```python
from build123d import *

# Parameters (mm, degrees)
SKETCH1_R           = 6.5
BOSS_EXTRUDE1_DEPTH = 3.5
SKETCH2_R           = 2
CUT_EXTRUDE1_DEPTH  = 10
CUT_EXTRUDE2_START  = -3.5
CUT_EXTRUDE2_DEPTH  = 1


with BuildPart() as part:
    # Sketch1 → Boss-Extrude1 (new body)
    with BuildSketch(Plane.XY):
        with BuildLine():
            Line((-15, 0), (-22.911315665, -21.736161147))
            ThreePointArc((-22.911315665, -21.736161147), (-25.84024514, -25.553216354), (-30.428856631, -27))
            Line((-30.428856631, -27), (-35, -27))
            Line((-35, -27), (-35, -35))
            Line((-35, -35), (35, -35))
            Line((35, -35), (35, -27))
            Line((35, -27), (30.428856631, -27))
            ThreePointArc((30.428856631, -27), (25.84024514, -25.553216354), (22.911315665, -21.736161147))
            Line((22.911315665, -21.736161147), (15, 0))
            ThreePointArc((15, 0), (0, 15), (-15, 0))
        make_face()
        Circle(SKETCH1_R, mode=Mode.SUBTRACT)
    extrude(amount=BOSS_EXTRUDE1_DEPTH)

    # Sketch2 → Cut-Extrude1 (cut)
    with BuildSketch(Plane.XY.offset(3.5)):
        with Locations((-14.142135624, -14.142135624)):
            Circle(SKETCH2_R)
        with Locations((0, -20)):
            Circle(SKETCH2_R)
        with Locations((14.142135624, -14.142135624)):
            Circle(SKETCH2_R)
    extrude(amount=-CUT_EXTRUDE1_DEPTH, mode=Mode.SUBTRACT)

    # Sketch3 → Cut-Extrude2 (cut)
    with BuildSketch(Plane(origin=(0, 0, 0), x_dir=(-1, 0, 0), z_dir=(0, 0, -1)).offset(CUT_EXTRUDE2_START)):
        with BuildLine():
            Line((-12.404038948, -11.696932167), (-12.02081528, -11.313708499))
            Line((-12.02081528, -11.313708499), (-11.313708499, -12.02081528))
            Line((-11.313708499, -12.02081528), (-11.696932167, -12.404038948))
            ThreePointArc((-11.696932167, -12.404038948), (-16.263455967, -16.263455967), (-12.404038948, -11.696932167))
        make_face()
        with BuildLine():
            Line((-0.5, -17.041960108), (-0.5, -16.5))
            Line((-0.5, -16.5), (0.5, -16.5))
            Line((0.5, -16.5), (0.5, -17.041960108))
            ThreePointArc((0.5, -17.041960108), (0, -23), (-0.5, -17.041960108))
        make_face()
        with BuildLine():
            Line((11.696932167, -12.404038948), (11.313708499, -12.02081528))
            Line((11.313708499, -12.02081528), (12.02081528, -11.313708499))
            Line((12.02081528, -11.313708499), (12.404038948, -11.696932167))
            ThreePointArc((12.404038948, -11.696932167), (16.263455967, -16.263455967), (11.696932167, -12.404038948))
        make_face()
    extrude(amount=CUT_EXTRUDE2_DEPTH, mode=Mode.SUBTRACT)


solid = part.part
```
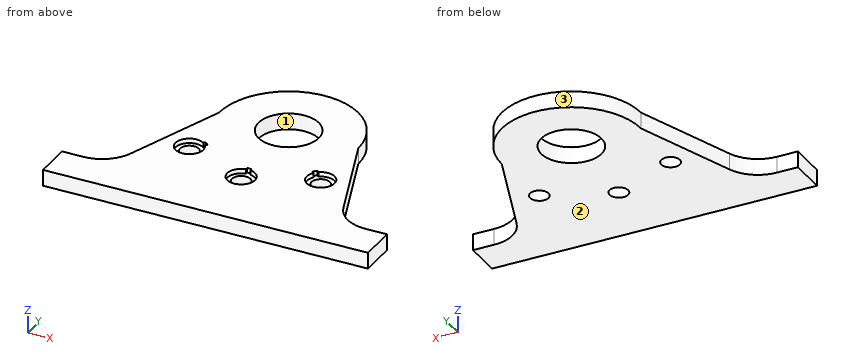
Can you work these out from the model? Positions are in its coordinate system, mm. Face numbers are marked on the shaded views. Give positions to 0.01 mm unless a question says otherwise; leave off trailing zeros. Order: outer loops, then holes, each group sorted by start corner. A loop starts at its lowest first (then second) coordinate and runs counter-clockwise, first axis right, second up. Notation, with made-up numbers: M -34,33.5 L 5,33.5 A31 ccw 5,62.5 Z; hole C -32.5,79.25 d9. An arc over 180 degrees is marked long. One line per item, written item: value.
1) We'd pull the mould along Y, two halves only. Please class the marked faces 1, 2 and 3: released by +Y, released by -Y, zero draft, split by the parting line, or undercut.
Answer sheet:
face 1: undercut
face 2: zero draft
face 3: released by +Y
2) I want a section at B-B, the plane z = 0.75. List the corners of the cut face in (x, y) for me, plus the area to 3 significant figures.
Answer sheet:
outline: M -35,-35 L 35,-35 L 35,-27 L 30.43,-27 A8 cw 22.91,-21.74 L 15,0 A15 ccw -15,0 L -22.91,-21.74 A8 cw -30.43,-27 L -35,-27 Z; hole C -14.14,-14.14 d4; hole C 0,0 d13; hole C 0,-20 d4; hole C 14.14,-14.14 d4
area: 1,830 mm^2
3) For P1, Ø6.5, axis at x = -14.14, y = -14.14, coming from the +Z side; P2, Ø4.5, axis at x = 0, y = -20, coming from the +Z side; P3, Ø1.5, axis at y = 0, z = 0.5, coming from the +X side; P4, Ø2, axis at y = -3.5, z = 1, coming from the -X side, each with a flat end and sliding along its axis, tell me the tip position at first contact or that it passes through.
Answer sheet:
P1: stops at z = 3.5
P2: stops at z = 2.5
P3: stops at x = 15.27
P4: stops at x = -16.64
4) I want a section at D-D, the plane y = 10. List the corners of the cut face in (x, z) for me.
Answer sheet:
outline: M -11.18,0 L 11.18,0 L 11.18,3.5 L -11.18,3.5 Z
5) I want a section at C-C, the plane x = 29. List the corners of the cut face in (y, z) for me.
Answer sheet:
outline: M -35,0 L -26.87,0 L -26.87,3.5 L -35,3.5 Z
6) I want a section at A-A, the plane y = -20. List the corners of the cut face in (x, z) for me, plus the area to 3 significant figures.
Answer sheet:
outline: M -22.28,0 L -2,0 L -2,2.5 L -3,2.5 L -3,3.5 L -22.28,3.5 Z; M 2,0 L 22.28,0 L 22.28,3.5 L 3,3.5 L 3,2.5 L 2,2.5 Z
area: 140 mm^2
7) Please list where these lines run through material, in increasing order: line 1 along Y through (x, z) = (0, 1.95); line 2 along Y through (x, z) = (0, 2.9); line 3 along Y through (x, z) = (-4.5, 1.3).
Answer sheet:
line 1: y = -35 to -22, -18 to -6.5, 6.5 to 15
line 2: y = -35 to -23, -16.5 to -6.5, 6.5 to 15
line 3: y = -35 to -4.69, 4.69 to 14.31
